Design review of the part built by this model. Coordinates are the model's own, in mm. Coordinates: 2 decimals unless noted, no trailing zeros. Loops run counter-clockwise (first coordinate to the right, second up) from the corner with the lowest first, then second, coordinate; pieces in that order, holes last. Notation, with made-up numbers: (41, -14.75) -> (69, -14.75) arc R21 ccw to (69, 0.25) -> close; hole circle Ø8 at (54.5, 2). An arc over 180 degrees is marked (long way). Use one line per item in the form item = value. Start each with the question number.
1. Wall thickness on line 1 (Z direction, x = -13, y = 16); line 2 (Z direction, x = -13.5, y = 29); line 3 (X direction, y = 3.5, z = 40.5): over which ranges is each line inside the solid? List them lowest first. Write a range as from..to.
2. Consider section B-B (z = 25.4). State the section outline as (x, y) points, then the cut area to 3 significant figures.
3. Consider section A-A (y = 28.5). State how many separate pieces and enclosed holes the cut face has, then the cut area to 3 significant figures.
4. Consider section C-C (y = 9). State the section outline as (x, z) points (3 decimals).
5. Consider section D-D (x = 27.5). State the section outline as (y, z) points (3 decimals), then the cut area to 3 significant figures.
6. For pin 1 (4 mm diameter, centred on x = 28.3, y = 27.61, fed in from +Z); pin 2 (5.5 mm diameter, centred on x = 5.44, z = 44.45, fed in from -Y), all flat-tipped, find the tip position at first contact; note any pin that passes through.
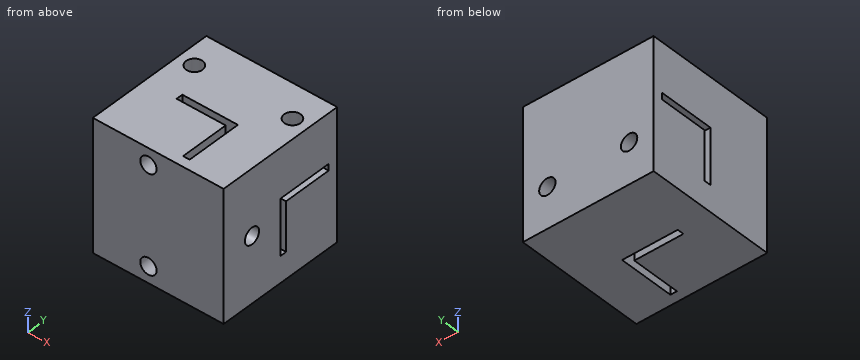
from build123d import *

# Parameters (mm, degrees)
F0_W      = 50.8
F0_H      = 50.8
F1_DEPTH  = 50.8
F3_DEPTH  = 50.8
F5_DEPTH  = 50.8
F6_R      = 3.175
F7_DEPTH  = 22.86
F8_R      = 3.175
F9_DEPTH  = 16.51
F10_R     = 3.175
F11_DEPTH = 19.05
F12_R     = 3.175
F13_DEPTH = 22.86


with BuildPart() as f1:
    # F0 (on Top) → F1 (new body)
    with BuildSketch(Plane.XY):
        with Locations((9.251333, 14.910408)):
            Rectangle(F0_W, F0_H)
    extrude(amount=F1_DEPTH)

    # F2 (on face) → F3 (cut, through all)
    with BuildSketch(Plane.XY.offset(50.8)):
        Polygon((-3.448667, 14.910408), (-3.448667, 12.370408), (15.601333, 12.370408), (15.601333, -6.679592), (18.141333, -6.679592), (18.141333, 14.910408), align=None)
    extrude(amount=-F3_DEPTH, mode=Mode.SUBTRACT)

    # F4 (on face) → F5 (cut, through all)
    with BuildSketch(Plane(origin=(-16.148667, 0, 0), x_dir=(0, -1, 0), z_dir=(-1, 0, 0))):
        Polygon((-14.910408, 10.16), (-14.910408, 31.75), (-36.500408, 31.75), (-36.500408, 29.21), (-17.450408, 29.21), (-17.450408, 10.16), align=None)
    extrude(amount=-F5_DEPTH, mode=Mode.SUBTRACT)

    # F6 (on face) → F7 (cut, through all)
    with BuildSketch(Plane.XZ.offset(10.489592)):
        with Locations((5.441333, 44.45)):
            Circle(F6_R)
        with Locations((5.441333, 6.35)):
            Circle(F6_R)
    extrude(amount=-F7_DEPTH, mode=Mode.SUBTRACT)

    # F8 (on face) → F9 (cut, through all)
    with BuildSketch(Plane.YZ.offset(34.651333)):
        with Locations((2.210408, 25.4)):
            Circle(F8_R)
    extrude(amount=-F9_DEPTH, mode=Mode.SUBTRACT)

    # F10 (on face) → F11 (cut, through all)
    with BuildSketch(Plane.XY.offset(50.8)):
        with Locations((28.301333, 27.610408)):
            Circle(F10_R)
        with Locations((-9.798667, 27.610408)):
            Circle(F10_R)
    extrude(amount=-F11_DEPTH, mode=Mode.SUBTRACT)

    # F12 (on face) → F13 (cut, through all)
    with BuildSketch(Plane(origin=(0, 40.310408, 0), x_dir=(-1, 0, 0), z_dir=(0, 1, 0))):
        with Locations((-25.126333, 15.875)):
            Circle(F12_R)
        with Locations((6.623667, 15.875)):
            Circle(F12_R)
    extrude(amount=-F13_DEPTH, mode=Mode.SUBTRACT)


solid = f1.part
Geometry check:
q1.line_1 = 0..10.16, 31.75..50.8
q1.line_2 = 0..29.21, 31.75..50.8
q1.line_3 = -16.15..15.6, 18.14..34.65
q2.outline = (-16.15, -10.49) -> (34.65, -10.49) -> (34.65, -0.96) -> (18.14, -0.96) -> (18.14, -6.68) -> (15.6, -6.68) -> (15.6, 12.37) -> (-3.45, 12.37) -> (-3.45, 14.91) -> (-16.15, 14.91) -> close; (-16.15, 17.45) -> (34.65, 17.45) -> (34.65, 40.31) -> (-16.15, 40.31) -> close; (18.14, 5.39) -> (34.65, 5.39) -> (34.65, 14.91) -> (18.14, 14.91) -> close
q2.area = 2,240 mm²
q3.separate_pieces = 4
q3.enclosed_holes = 2
q3.area = 2,160 mm²
q4.outline = (-16.149, 0) -> (15.601, 0) -> (15.601, 50.8) -> (-16.149, 50.8) -> close; (18.141, 0) -> (34.651, 0) -> (34.651, 50.8) -> (18.141, 50.8) -> close; hole circle Ø6.35 at (5.441, 6.35); hole circle Ø6.35 at (5.441, 44.45)
q5.outline = (-10.49, 0) -> (40.31, 0) -> (40.31, 13.766) -> (17.45, 13.766) -> (17.45, 10.16) -> (14.91, 10.16) -> (14.91, 31.75) -> (24.538, 31.75) -> (24.538, 50.8) -> (-10.49, 50.8) -> close; (17.45, 17.984) -> (40.31, 17.984) -> (40.31, 50.8) -> (30.683, 50.8) -> (30.683, 31.75) -> (36.5, 31.75) -> (36.5, 29.21) -> (17.45, 29.21) -> close; hole circle Ø6.35 at (2.21, 25.4)
q5.area = 2,230 mm²
q6.pin_1 = 29.21
q6.pin_2 = 14.91
